Here's how the part is built. I have some questions about the finished solid (model axes, mm). Face numbers are marked on the shaded views. A direction names the side the tool comes from. Give positions to 0.01 mm unless a question says otherwise; leave off trailing zeros. Order: outer loops, then holes, each group sorted by start corner. A loop starts at its lowest first (then second) coordinate and runs counter-clockwise, first axis right, second up. Notation, with made-up numbers: (-25, 38.25) -> (26, 38.25) arc R23 cw to (26, 59.25) -> close; hole circle Ø6 at (-31, 58.25). An arc over 180 degrees is marked (long way). Write each question's results on one line, items separated by ' | '. Start each with the question number.
Q1. For the marked faces 1, 2 and 3, which set-ups out of +Z, -Z, +X, -X, +Y, -Y let a thin tool reach every point of the face, with its end or its side?
Q2. Imagine slicing it at B-B, the plane y = 9.25. Please give me the cut outline in (x, z), then the cut area to 3 significant figures.
Q3. Imagine slicing it at A-A, the plane x = 0. Please give me the cut outline in (y, z), then the cut area to 3 significant figures.
Q4. I need wall thicknesses on line 1 along X through (y, z) = (1, -22); line 2 along Z through (x, y) = (-25, 1.75); line 3 along X through (y, z) = (4.25, 36.5). Which ranges of each line are inside material? Lowest first, please. Write a range as [from, to].
Q5. Imagine slicing it at C-C, the plane y = 3.75. State how many separate pieces and enclosed holes the cut face has, then the cut area to 3 significant figures.
Q6. I'm going to push flat-ended pins straight in: pin 1 (5 mm diameter, centred on x = -3.5, y = 3, fed in from -Z); pin 2 (1 mm diameter, centred on y = 7, z = 3.5, fed in from -X); pin 3 (10 mm diameter, centred on x = 39.5, z = -7.5, fed in from +Y); pin 4 (2 mm diameter, centred on x = -41.5, z = -8, fed in from -Y). Where does each tip first touch, or does it pass through?
```python
from build123d import *

# Parameters (mm, degrees)
SKETCH1_R           = 50.5
BOSS_EXTRUDE1_DEPTH = 5
SKETCH2_R           = 8.5
SKETCH2_R_2         = 1.25
CUT_EXTRUDE1_DEPTH  = 72.592597383
CIRPATTERN1_COUNT   = 4
SKETCH3_R           = 1.75
BOSS_EXTRUDE2_DEPTH = 10
FILLET2_R           = 3
SKETCH4_R           = 1.7
SKETCH4_R_2         = 3.2639
CUT_EXTRUDE2_DEPTH  = 73.114492302
SKETCH7_R           = 4.5
CUT_EXTRUDE9_DEPTH  = 73.97602346
SKETCH8_R           = 1.7
CUT_EXTRUDE10_DEPTH = 73.97602346
CIRPATTERN2_COUNT   = 4


with BuildPart() as part:
    # Sketch1 → Boss-Extrude1 (new body)
    with BuildSketch(Plane(origin=(0, 0, 0), x_dir=(1, 0, 0), z_dir=(0, 1, 0))):
        with Locations(Location((0, 0, 0), (0, 0, 270))):
            Circle(SKETCH1_R)
    extrude(amount=BOSS_EXTRUDE1_DEPTH)

    # Sketch2 → Cut-Extrude1 (cut, through all)
    with BuildSketch(Plane(origin=(0, 5, 0), x_dir=(1, 0, 0), z_dir=(0, 1, 0))):
        with Locations(Location((34, 0, 0), (0, 0, 270))):
            Circle(SKETCH2_R)
        with Locations(Location((41.5, -8, 0), (0, 0, 270))):
            Circle(SKETCH2_R_2)
        with Locations(Location((41.5, 8, 0), (0, 0, 270))):
            Circle(SKETCH2_R_2)
        with Locations(Location((11.5, 8, 0), (0, 0, 270))):
            Circle(SKETCH2_R_2)
        with Locations(Location((11.5, -8, 0), (0, 0, 270))):
            Circle(SKETCH2_R_2)
    cut_extrude1 = extrude(amount=-CUT_EXTRUDE1_DEPTH, mode=Mode.SUBTRACT)

    # CirPattern1: Cut-Extrude1 ×4 about axis
    cirpattern1_axis = Axis((0, 0, 0), (0, 1, 0))
    for i in range(1, CIRPATTERN1_COUNT):
        add(cut_extrude1.rotate(cirpattern1_axis, i * 360 / CIRPATTERN1_COUNT), mode=Mode.SUBTRACT)

    # Sketch3 → Boss-Extrude2 (add)
    with BuildSketch(Plane(origin=(0, 5, 0), x_dir=(1, 0, 0), z_dir=(0, 1, 0))):
        Polygon((0, -14.849242405), (14.849242405, 0), (0, 14.849242405), (-14.849242405, 0), align=None)
        with Locations(Location((10, 0, 0), (0, 0, 270))):
            Circle(SKETCH3_R, mode=Mode.SUBTRACT)
        with Locations(Location((0, -10, 0), (0, 0, 270))):
            Circle(SKETCH3_R, mode=Mode.SUBTRACT)
        with Locations(Location((-10, 0, 0), (0, 0, 270))):
            Circle(SKETCH3_R, mode=Mode.SUBTRACT)
        with Locations(Location((0, 10, 0), (0, 0, 270))):
            Circle(SKETCH3_R, mode=Mode.SUBTRACT)
    extrude(amount=BOSS_EXTRUDE2_DEPTH)

    # Fillet2
    fillet2_edges = [part.edges().sort_by_distance(p)[0] for p in [
        (-14.849242405, 10, 0),
        (0, 10, 14.849242405),
        (14.849242405, 10, 0),
        (0, 10, -14.849242405),
    ]]
    fillet(fillet2_edges, radius=FILLET2_R)

    # Sketch4 → Cut-Extrude2 (cut, through all)
    with BuildSketch(Plane(origin=(0, 5, 0), x_dir=(1, 0, 0), z_dir=(0, 1, 0))):
        with Locations(Location((21.213203436, 21.213203436, 0), (0, 0, 270))):
            Circle(SKETCH4_R)
        with Locations(Location((-21.213203436, -21.213203436, 0), (0, 0, 90))):
            Circle(SKETCH4_R)
        with Locations(Location((-24.748737342, 24.748737342, 0), (0, 0, 270))):
            Circle(SKETCH4_R_2)
        with Locations(Location((24.748737342, -24.748737342, 0), (0, 0, 90))):
            Circle(SKETCH4_R_2)
        with Locations(Location((15.556349186, 15.556349186, 0), (0, 0, 270))):
            Circle(SKETCH4_R)
        with Locations(Location((-15.556349186, -15.556349186, 0), (0, 0, 90))):
            Circle(SKETCH4_R)
        Polygon((20.859650045, 28.637824638), (29.344931419, 37.123106012), (26.516504294, 39.951533137), (18.03122292, 31.466251763), align=None)
        Polygon((31.466251763, 18.03122292), (39.951533137, 26.516504294), (37.123106012, 29.344931419), (28.637824638, 20.859650045), align=None)
        Polygon((-26.516504294, -39.951533137), (-29.344931419, -37.123106012), (-20.859650045, -28.637824638), (-18.03122292, -31.466251763), align=None)
        Polygon((-37.123106012, -29.344931419), (-39.951533137, -26.516504294), (-31.466251763, -18.03122292), (-28.637824638, -20.859650045), align=None)
    extrude(amount=-CUT_EXTRUDE2_DEPTH, mode=Mode.SUBTRACT)

    # Sketch7 → Cut-Extrude9 (cut, through all)
    with BuildSketch(Plane(origin=(0, 0, 0), x_dir=(1, 0, 0), z_dir=(0, 1, 0))):
        with Locations(Location((-37.314116231, 23.316447626, 0), (0, 0, 270))):
            Circle(SKETCH7_R)
    extrude(amount=CUT_EXTRUDE9_DEPTH, mode=Mode.SUBTRACT)

    # Sketch8 → Cut-Extrude10 (cut, through all)
    with BuildSketch(Plane(origin=(0, 0, 0), x_dir=(1, 0, 0), z_dir=(0, 1, 0))):
        with Locations(Location((-15.561916521, 42.756014246, 0), (0, 0, 270))):
            Circle(SKETCH8_R)
        with Locations(Location((15.561916521, 42.756014246, 0), (0, 0, 270))):
            Circle(SKETCH8_R)
    cut_extrude10 = extrude(amount=CUT_EXTRUDE10_DEPTH, mode=Mode.SUBTRACT)

    # CirPattern2: Cut-Extrude10 ×4 about axis
    cirpattern2_axis = Axis((0, 0, 0), (0, 1, 0))
    for i in range(1, CIRPATTERN2_COUNT):
        add(cut_extrude10.rotate(cirpattern2_axis, i * 360 / CIRPATTERN2_COUNT), mode=Mode.SUBTRACT)


solid = part.part
```
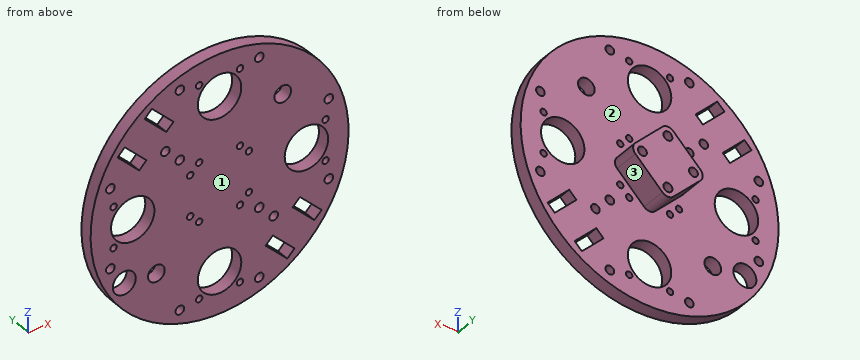
Geometry check:
1) face 1: +Z, -Z, +X, -X, -Y | face 2: +Y | face 3: -Z, +X, +Y
2) outline: (-12.73, -2.12) -> (-2.12, -12.73) arc R3 ccw to (2.12, -12.73) -> (12.73, -2.12) arc R3 ccw to (12.73, 2.12) -> (2.12, 12.73) arc R3 ccw to (-2.12, 12.73) -> (-12.73, 2.12) arc R3 ccw to start; hole circle Ø3.5 at (-10, 0); hole circle Ø3.5 at (0, -10); hole circle Ø3.5 at (0, 10); hole circle Ø3.5 at (10, 0) | area: 395 mm²
3) outline: (0, -50.5) -> (5, -50.5) -> (5, -42.5) -> (0, -42.5) -> close; (0, -25.5) -> (5, -25.5) -> (5, -13.61) -> (15, -13.61) -> (15, -11.75) -> (5, -11.75) -> (5, -8.25) -> (15, -8.25) -> (15, 8.25) -> (5, 8.25) -> (5, 11.75) -> (15, 11.75) -> (15, 13.61) -> (5, 13.61) -> (5, 25.5) -> (0, 25.5) -> close; (0, 42.5) -> (5, 42.5) -> (5, 50.5) -> (0, 50.5) -> close | area: 537 mm²
4) line 1: [-45.46, -41.62], [-33.01, -26.51], [-22.99, 19.71], [22.72, 29.78], [35.44, 45.46] | line 2: [-43.88, -28], [-21.49, 32.78], [38.44, 43.88] | line 3: [-34.9, -28.72], [-23.06, -8.12], [8.12, 34.9]
5) separate pieces: 1 | enclosed holes: 39 | area: 6,590 mm²
6) pin 1: z = -50.49 | pin 2: x = -11.85 | pin 3: y = 5 | pin 4: through
